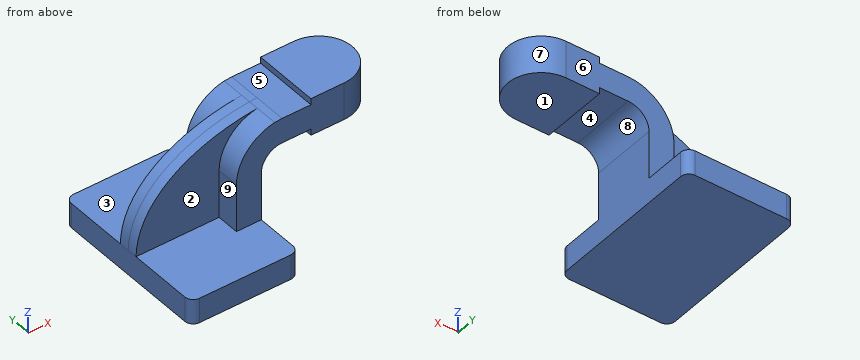
from build123d import *

# Parameters (mm, degrees)
F1_DEPTH = 63.5
F2_DEPTH = 25.4
F3_DEPTH = 7.9375
F0_W     = 25.4
F0_H     = 28.575
F5_R     = 6.35


with BuildPart() as f1:
    # F0 (on Front) → F1 (new body, symmetric)
    with BuildSketch(Plane.XZ):
        Polygon((-41.275, 9.525), (-41.275, -9.525), (41.275, -9.525), (41.275, 9.525), (22.224999, 9.525), align=None)
    extrude(amount=F1_DEPTH, both=True)

    # F0 (on Front) → F2 (join, symmetric)
    with BuildSketch(Plane.XZ):
        with BuildLine():
            Line((22.224999, 9.525), (41.275, 9.525))
            Line((41.275, 9.525), (41.275, 46.0502))
            ThreePointArc((41.275, 46.0502), (45.92468, 57.27552), (57.15, 61.9252))
            Line((57.15, 61.9252), (79.210615, 61.9252))
            Line((79.210615, 61.9252), (79.210615, 80.975201))
            Line((79.210615, 80.975201), (57.15, 80.975201))
            add(Edge.make_bspline(
                [(51.463786, 80.5092), (53.33983, 80.690444), (55.23552, 80.845904), (57.15, 80.975201)],
                knots=[117.550544, 117.550544, 117.550544, 117.550544, 121.624882, 121.624882, 121.624882, 121.624882], degree=3))
            ThreePointArc((51.463786, 80.5092), (30.519691, 68.646269), (22.224999, 46.0502))
            Line((22.224999, 46.0502), (22.224999, 9.525))
        make_face()
        Polygon((79.210615, 85.725), (79.210615, 80.975201), (79.210615, 61.9252), (79.210615, 57.15), (104.610615, 57.15), (104.610615, 85.725), align=None)
    extrude(amount=F2_DEPTH, both=True)

    # F0 (on Front) → F3 (join, symmetric)
    with BuildSketch(Plane.XZ):
        with BuildLine():
            add(Edge.make_bspline(
                [(-41.275, 9.525), (-40.4355, 48.588255), (-2.662796, 75.280054), (51.463786, 80.5092)],
                knots=[0, 0, 0, 0, 117.550544, 117.550544, 117.550544, 117.550544], degree=3))
            Line((-41.275, 9.525), (22.224999, 9.525))
            Line((22.224999, 9.525), (22.224999, 46.0502))
            ThreePointArc((22.224999, 46.0502), (30.519691, 68.646269), (51.463786, 80.5092))
        make_face()
    extrude(amount=F3_DEPTH, both=True)

    # F0 (on Front) → F4 (revolve)
    with BuildSketch(Plane.XZ):
        with Locations((117.310615, 71.4375)):
            Rectangle(F0_W, F0_H)
    revolve(axis=Axis((104.610615, 0, 71.4375), (0, 0, 1)))

    # F5
    f5_edges = [f1.edges().sort_by_distance(p)[0] for p in [
        (41.275, -63.5, 0),
        (41.275, 63.5, 0),
        (-41.275, 63.5, 0),
        (-41.275, -63.5, 0),
    ]]
    fillet(f5_edges, radius=F5_R)


solid = f1.part
Can you work these out from the model? Positions are in its coordinate system, mm. Face numbers are marked on the shaded views. A direction names the side the tool comes from. Coordinates: 2 decimals unless noted, no trailing zeros. Order: outer loops, then holes, each group sorted by start corner. A loop starts at its lowest first (then second) coordinate and runs counter-clockwise, first axis right, second up. Notation, with made-up numbers: (-39.5, 48) -> (-12.5, 48) arc R29 cw to (-12.5, 83) -> close; hole circle Ø10 at (-1.75, 72.25). An arc over 180 degrees is marked (long way). Use one line per item in the form item = value.
Q1. We'd pull the mould along X, two halves only. Please class the marked faces 6, 7, 8 and 9: released by +X, released by -X, zero draft, split by the parting line, or undercut.
From the geometry:
face_6 = zero draft
face_7 = released by +X
face_8 = undercut
face_9 = released by -X
Q2. Will these pins go through, and if not, where does the flat tip stop? P1, Ø4, axis at x = -12.5, y = 15.5, coming from the +Z side (3 decimals); P2, Ø8.5, axis at y = -16, z = 30.5, coming from the -X side (3 decimals); P3, Ø16.5, axis at y = 23.5, z = 20.5, coming from the +X side (3 decimals).
From the geometry:
P1 = 9.525
P2 = 22.225
P3 = 41.275
Q3. Imagine slicing it at B-B, the plane x = 97. List the corners of the cut face in (y, z) for me (3 decimals), then the cut area to 3 significant figures.
From the geometry:
outline = (-25.4, 57.15) -> (25.4, 57.15) -> (25.4, 85.725) -> (-25.4, 85.725) -> close
area = 1,450 mm²
Q4. Which directions (+Z, -Z, +X, -X, +Y, -Y) give clear straight access to the entire face, cutting with the end or side of a thin tool? Please do the marked faces 1, 2, 3, 4 and 5.
From the geometry:
face_1 = -Z, +X, +Y, -Y
face_2 = +Z, -X, -Y
face_3 = +Z, -X, +Y
face_4 = -Z, +Y, -Y
face_5 = +Z, -X, +Y, -Y
Q5. Imagine slicing it at A-A, the plane y = -47. List the corners of the cut face in (x, z) for me (3 decimals).
From the geometry:
outline = (-41.275, -9.525) -> (41.275, -9.525) -> (41.275, 9.525) -> (-41.275, 9.525) -> close
Q6. I need wall thicknesses on L1, parallel to Y at x = -8, z = 39; L2, parallel to X at y = -20.5, z = 9 (3 decimals); L3, parallel to Z at x = 60.5, y = -6. Which ranges of each line are inside material? Lowest first, please.
From the geometry:
L1 = -7.94 to 7.94
L2 = -41.275 to 41.275
L3 = 61.93 to 80.98
